```python
from build123d import *

# Parameters (mm, degrees)
F0_W     = 15
F0_H     = 15
F1_DEPTH = 15
F2_R     = 5.25
F3_DEPTH = 10
F4_R     = 5.5
F4_R_2   = 5.25
F5_DEPTH = 2


with BuildPart() as f1:
    # F0 (on Front) → F1 (new body)
    with BuildSketch(Plane.XZ):
        Rectangle(F0_W, F0_H)
    extrude(amount=F1_DEPTH)

    # F2 (on face) → F3 (cut)
    with BuildSketch(Plane.XZ.offset(15)):
        Circle(F2_R)
    extrude(amount=-F3_DEPTH, mode=Mode.SUBTRACT)

    # F4 (on face) → F5 (cut)
    with BuildSketch(Plane.XZ.offset(5)):
        Circle(F4_R)
        Circle(F4_R_2, mode=Mode.SUBTRACT)
    extrude(amount=F5_DEPTH, mode=Mode.SUBTRACT)


solid = f1.part
```
Can you work these out from the model? Positions are in its coordinate system, mm. A direction names the side the tool comes from. Coordinates: 2 decimals unless noted, no trailing zeros. Loops run counter-clockwise (first coordinate to the right, second up) from the corner with the lowest first, then second, coordinate; pieces in that order, holes last.
Item 1: Please list where these lines run through material, in increasing order: L1, parallel to Z at x = 0, y = -12.25; L2, parallel to Z at x = 0, y = -6.5; L3, parallel to Y at x = 1.25, z = 0.75.
Answers below:
L1: z = -7.5 to -5.25, 5.25 to 7.5
L2: z = -7.5 to -5.5, 5.5 to 7.5
L3: y = -5 to 0
Item 2: Suppose I cut it at B-B (y = -11.5). Please give me the cut outline in (x, z).
Answers below:
outline: (-7.5, -7.5) - (7.5, -7.5) - (7.5, 7.5) - (-7.5, 7.5) - close; hole circle Ø10.5 at (0, 0)
Item 3: Suppose I cut it at A-A (x = 0). Please give me the cut outline in (y, z).
Answers below:
outline: (-15, -7.5) - (0, -7.5) - (0, 7.5) - (-15, 7.5) - (-15, 5.25) - (-7, 5.25) - (-7, 5.5) - (-5, 5.5) - (-5, -5.5) - (-7, -5.5) - (-7, -5.25) - (-15, -5.25) - close
Item 4: If we mould it in two halves opening along X, with no side actions, what happens to faces 4 (the face through (-7.5, -7, 0)), 5 (the face through (0, -5, 0)), 6 (the face through (0, 0, 0))? For each: released by +X, released by -X, zero draft, split by the parting line, or undercut.
Answers below:
face 4: released by -X
face 5: undercut
face 6: zero draft
Item 5: Suppose I cut it at C-C (z = 0). Please give me the cut outline in (x, y), then the cut area to 3 significant figures.
Answers below:
outline: (-7.5, -15) - (-5.25, -15) - (-5.25, -7) - (-5.5, -7) - (-5.5, -5) - (5.5, -5) - (5.5, -7) - (5.25, -7) - (5.25, -15) - (7.5, -15) - (7.5, 0) - (-7.5, 0) - close
area: 119 mm2
Item 6: Which directions (+Z, -Z, +X, -X, +Y, -Y) give clear straight access to the entire face, cutting with the end or side of a thin tool? Please do faces 1 (the face through (-1.19, -5.99, -5.37)), 2 (the face through (5, -11.1, 1.6)), 3 (the face through (0, -7, 7.5)).
Answers below:
face 1: none
face 2: -Y
face 3: +Z, +X, -X, +Y, -Y
